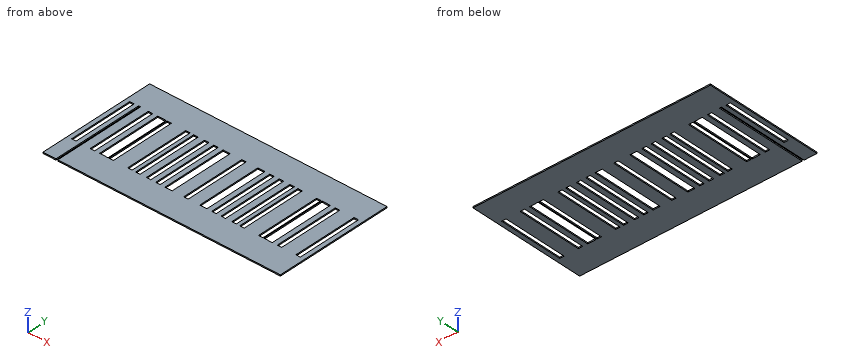
Autodesk Inventor part; units mm, degrees
ref_plane "acrylic_sheet_plane" through (0, 0, 4) normal (0, 0, 1) x (1, 0, 0)
ref_plane "YZ Plane" through (0, 0, 0) normal (1, 0, 0) x (0, 1, 0)
ref_plane "XZ Plane" through (0, 0, 0) normal (0, 1, 0) x (-1, 0, 0)
sketch "ferrite_layer_outline_sketch" plane through (0, 0, 0) normal (0, 0, 1) x (1, 0, 0)
  line L0 (0, 200) -> (800, 200)
  line L1 (800, 200) -> (800, -200)
  line L2 (800, -200) -> (0, -200)
  line L3 (0, -200) -> (0, 200)
  line L4 (-160, 0) -> (960, 0)
  line L5 (400, 200) -> (400, -200) construction
  line L6 (400, 366.8869) -> (400, -324.3455) construction
  line L7 (400, 200) -> (400, -200)
  point P0 (0, 0)
  point P1 (0, 0)
  point P2 (0, 0)
  point P3 (0, 0)
  point P4 (20, 0)
  dimension "d0" = 800
  dimension "d1" = 400
extrude "Sheet Extrude" add sketch "ferrite_layer_outline_sketch" along normal blind 4
ref_plane "acrylic_sheet_plane" through (0, 0, 4) normal (0, 0, 1) x (1, 0, 0)
sketch "Sketch4" plane through (0, 0, 4) normal (0, 0, 1) x (1, 0, 0)
  line L0 (14.5, 109) -> (29.5, 109)
  line L1 (29.5, 109) -> (29.5, -109)
  line L2 (29.5, -109) -> (14.5, -109)
  line L3 (14.5, -109) -> (14.5, 109)
  line L4 (-12.6534, 0) -> (47.471, 0)
  line L5 (0, 200) -> (0, -200)
  line L6 (800, 200) -> (0, 200)
  line L7 (0, -200) -> (800, -200)
  point P0 (0, 0)
  point P1 (14.5, 0)
  point P2 (0, 0)
  dimension "d43" = 15
  dimension "d44" = 218
  dimension "d45" = 14.5
extrude "Extrusion9" cut sketch "Sketch4" against normal through all
pattern_linear "Rectangular Pattern 7 fer" count 7 spacing 126 along (1, 0, 0) of "Extrusion9"
pattern_linear "Rectangular Pattern 8 fer" count 8 spacing 108 along (1, 0, 0) of "Extrusion9"
pattern_linear "pattern_test_#_of_ferrites 9 fer" count 9 spacing 94.5 along (1, 0, 0) of "Extrusion9"
pattern_linear "Rectangular Pattern 10 fer" [suppressed]
pattern_linear "Rectangular Pattern 13" count 13 spacing 63 along (1, 0, 0) of "Extrusion9"
sketch "Sketch5" plane through (0, 0, 4) normal (0, 0, 1) x (1, 0, 0)
  line L0 (0, 200) -> (0, -200)
  line L1 (0, 150) -> (800, 150)
  line L2 (800, -200) -> (800, 200)
  line L3 (800, 200) -> (0, 200)
  line L4 (0, -200) -> (800, -200)
  line L5 (0, -150) -> (800, -150)
  point P0 (0, 0)
  dimension "d66" = 50
  dimension "d68" = 50
sketch "Sketch11" plane through (0, 0, 4) normal (0, 0, 1) x (1, 0, 0)
  circle A0 centre (47, 7.75) radius 3
  line L0 (800, 200) -> (0, 200)
  line L1 (0, 200) -> (0, -200)
  circle A1 centre (47, -72) radius 3
  line L2 (0, -200) -> (800, -200)
  point P0 (0, 0)
  dimension "d85" = 6
  dimension "d86" = 192.25
  dimension "d87" = 47
  dimension "d88" = 6
  dimension "d89" = 128
  dimension "d90" = 47
extrude "Extrusion15" cut sketch "Sketch11" against normal through all
sketch "Sketch12" plane through (0, 0, 4) normal (0, 0, 1) x (1, 0, 0)
  line L0 (0, -200) -> (800, -200)
  line L1 (43.5, 110.75) -> (50, 110.75)
  line L2 (50, 110.75) -> (50, -200)
  line L3 (50, -200) -> (43.5, -200)
  line L4 (43.5, -200) -> (43.5, 110.75)
  line L5 (0, 200) -> (0, -200)
  point P0 (0, 0)
  dimension "d97" = 310.75
  dimension "d98" = 6.5
  dimension "d99" = 43.5
extrude "Extrusion17" cut sketch "Sketch12" against normal through all
equation "\"d0\" = track_length"
equation "\"d1\" = track_width"
equation "\"d43\" = ferrite_width"
equation "\"d44\" = ferrite_length"
equation "\"d45\" = gap_distance"
equation "\"d50\" = parameter_5"
equation "\"d62\" = test_parameter_5"
equation "\"track_length\" = 800"
equation "\"track_width\" = 400"
equation "\"gap_distance\" = 14.5"
equation "\"ferrite_length\" = 218"
equation "\"ferrite_width\" = 15"
equation "\"ferrite_height\" = 8"
equation "\"acrylic_sheet_8mm\" = 8"
properties part number "ferrite_layer_dex_1R1"
Model file for the job. Use its own axes, mm. Round coordinates to 2 decimals unless told otherwise and drop trailing zeros. Loops run counter-clockwise (first coordinate to the right, second up) from the corner with the lowest first, then second, coordinate; pieces in that order, holes last.
1. Band-saw the part on B-B, the plane y = -59.5. Count the separate pieces of the cut face and the enclosed holes in it, and give its area (3 significant figures).
Check values:
separate pieces: 21
enclosed holes: 0
area: 1,850 mm2
2. Band-saw the part on A-A, the plane x = 461. List the corners of the cut face in (y, z), and give its area (3 significant figures).
Check values:
outline: (-200, 0) - (-109, 0) - (-109, 4) - (-200, 4) - close; (109, 0) - (200, 0) - (200, 4) - (109, 4) - close
area: 728 mm2
3. Wall check: probe 1 along X at (y, z) = (-116, 1.7); probe 2 along Y at (x, z) = (268, 3.35). Give the ranges that are in metal, low to high.
Check values:
probe 1: x = 0 to 43.5, 50 to 800
probe 2: y = -200 to -109, 109 to 200
